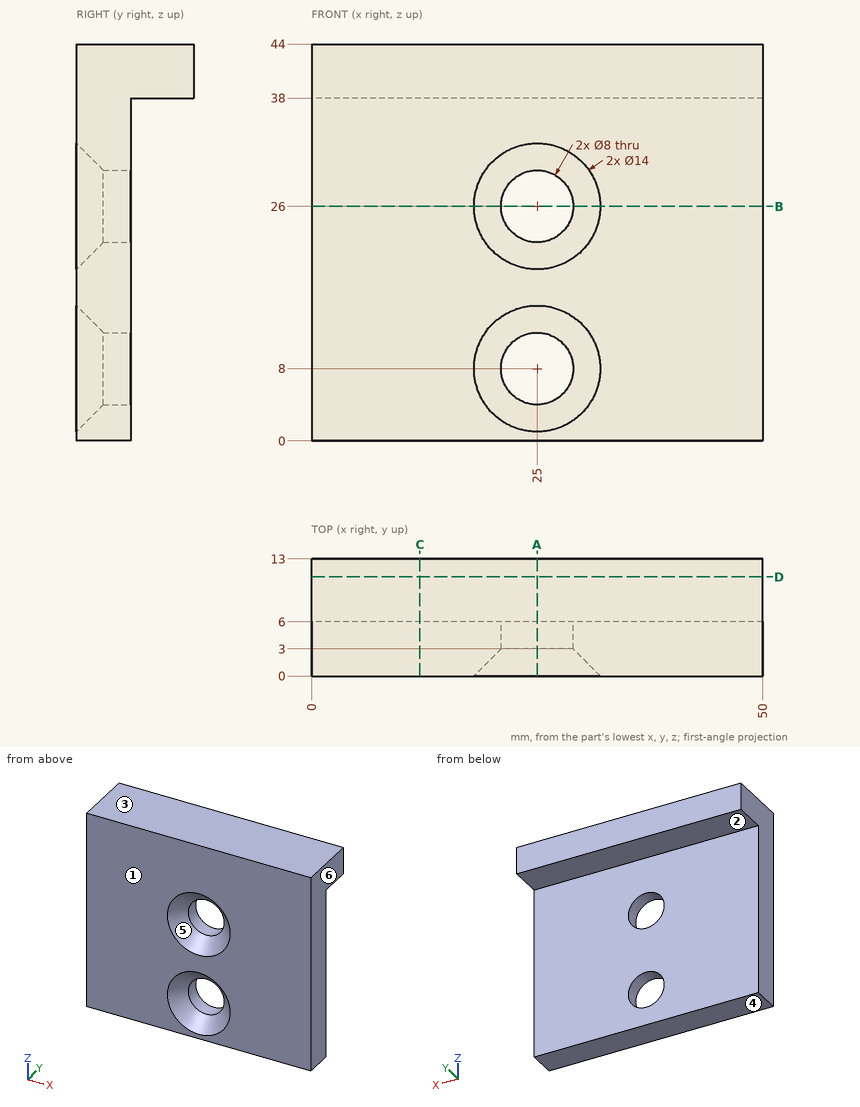
The drawing under review shows one solid part. Ordinate dimensions are in mm from its lowest x, y, z. A direction names the side the tool comes from. Round coordinates to 2 decimals unless told otherwise and drop trailing zeros. Write each loop counter-clockwise with the first axis right and the second up, starting at its lowest first coordinate (ties: lowest second). Pieces come first, ordered by that corner, then holes. Notation, with made-up numbers: M 39,44 L 50,44 A17 ccw 50,52 Z; hole C 72,64 d6. An arc over 180 degrees is marked long. One line per item, written item: value. Start each with the question number.
(1) We need section B-B (z = 26). Give the boundary of the cut face in (x, y).
(2) We need section A-A (x = 25). Give the boundary of the cut face in (y, z).
(3) Insertion check: pin 1 (9 mm diameter, centred on x = 25, z = 8, fed in from +Y); pin 2 (3.5 mm diameter, centred on x = 28.5, y = 10.5, fed in from -Z). Each pin has a flat end and moves straight along its axis. Give the tip position at first contact, or say it passes through.
(4) The part is to be moulded in two halves that separate along Z. For the marked faces 3, 4, 5 and 6, say which applies: released by +Z, released by -Z, zero draft, split by the parting line, or undercut.
(5) Machinability: for the marked faces 1 and 2, which of the approach directions +Z, -Z, +X, -X, +Y, -Y give a long, thin tool a straight path to every point of the face, cutting with its end or side? Answer none if there is none.
(6) Wall thickness on line 1 (Z direction, x = 25, y = 3.9); line 2 (X direction, y = 5.05, z = 8); line 3 (Z direction, x = 42, y = 10.75): over which ranges is each line inside the solid? List them lowest first.
(7) We need section D-D (y = 11). Give the boundary of the cut face in (x, z).
(8) We need section C-C (x = 12). Give the boundary of the cut face in (y, z).
Result:
1. outline: M 0,0 L 18,0 L 21,3 L 21,6 L 0,6 Z; M 29,3 L 32,0 L 50,0 L 50,6 L 29,6 Z
2. outline: M 0,0 L 6,0 L 6,4 L 3,4 L 0,1 Z; M 0,15 L 3,12 L 6,12 L 6,22 L 3,22 L 0,19 Z; M 0,33 L 3,30 L 6,30 L 6,38 L 13,38 L 13,44 L 0,44 Z
3. pin 1: y = 6
3. pin 2: z = 38
4. face 3: released by +Z
4. face 4: released by -Z
4. face 5: undercut
4. face 6: zero draft
5. face 1: +Z, -Z, +X, -X, -Y
5. face 2: -Z, +X, -X, +Y
6. line 1: 0 to 4, 12 to 22, 30 to 44
6. line 2: 0 to 21, 29 to 50
6. line 3: 38 to 44
7. outline: M 0,38 L 50,38 L 50,44 L 0,44 Z
8. outline: M 0,0 L 6,0 L 6,38 L 13,38 L 13,44 L 0,44 Z
